The model under review builds one solid part; all positions refer to its coordinate system, in mm. Give positions to 0.01 mm unless a question says otherwise; leave off trailing zeros. Order: outer loops, then holes, each group sorted by start corner. A loop starts at its lowest first (then second) coordinate and runs counter-clockwise, first axis right, second up.
```python
from build123d import *

# Parameters (mm, degrees)
SKETCH1_R           = 75
SKETCH1_R_2         = 5
BOSS_EXTRUDE1_DEPTH = 5


with BuildPart() as part:
    # Sketch1 → Boss-Extrude1 (new, symmetric)
    with BuildSketch(Plane.XY):
        Circle(SKETCH1_R)
        with Locations((62.5, 0)):
            Circle(SKETCH1_R_2, mode=Mode.SUBTRACT)
        with Locations((54.126587737, -31.25)):
            Circle(SKETCH1_R_2, mode=Mode.SUBTRACT)
        with Locations((31.25, -54.126587737)):
            Circle(SKETCH1_R_2, mode=Mode.SUBTRACT)
        with Locations((0, -62.5)):
            Circle(SKETCH1_R_2, mode=Mode.SUBTRACT)
        with Locations((-31.25, -54.126587737)):
            Circle(SKETCH1_R_2, mode=Mode.SUBTRACT)
        with Locations((-54.126587737, -31.25)):
            Circle(SKETCH1_R_2, mode=Mode.SUBTRACT)
        with Locations((-62.5, 0)):
            Circle(SKETCH1_R_2, mode=Mode.SUBTRACT)
        with Locations((-54.126587737, 31.25)):
            Circle(SKETCH1_R_2, mode=Mode.SUBTRACT)
        with Locations((-31.25, 54.126587737)):
            Circle(SKETCH1_R_2, mode=Mode.SUBTRACT)
        with Locations((0, 62.5)):
            Circle(SKETCH1_R_2, mode=Mode.SUBTRACT)
        with Locations((31.25, 54.126587737)):
            Circle(SKETCH1_R_2, mode=Mode.SUBTRACT)
        with Locations((54.126587737, 31.25)):
            Circle(SKETCH1_R_2, mode=Mode.SUBTRACT)
        with BuildLine():
            Line((45, 5), (46.314144708, 5))
            ThreePointArc((46.314144708, 5), (48.608912113, 6.067632914), (49.27036671, 8.510638298))
            ThreePointArc((49.27036671, 8.510638298), (35.355339059, 35.355339059), (8.510638298, 49.27036671))
            ThreePointArc((8.510638298, 49.27036671), (6.067632914, 48.608912113), (5, 46.314144708))
            Line((5, 46.314144708), (5, 45))
            Line((5, 45), (-5, 45))
            Line((-5, 45), (-5, 46.314144708))
            ThreePointArc((-5, 46.314144708), (-6.067632914, 48.608912113), (-8.510638298, 49.27036671))
            ThreePointArc((-8.510638298, 49.27036671), (-35.355339059, 35.355339059), (-49.27036671, 8.510638298))
            ThreePointArc((-49.27036671, 8.510638298), (-48.608912113, 6.067632914), (-46.314144708, 5))
            Line((-46.314144708, 5), (-45, 5))
            Line((-45, 5), (-45, -5))
            Line((-45, -5), (-46.314144708, -5))
            ThreePointArc((-46.314144708, -5), (-48.608912113, -6.067632914), (-49.27036671, -8.510638298))
            ThreePointArc((-49.27036671, -8.510638298), (-35.355339059, -35.355339059), (-8.510638298, -49.27036671))
            ThreePointArc((-8.510638298, -49.27036671), (-6.067632914, -48.608912113), (-5, -46.314144708))
            Line((-5, -46.314144708), (-5, -45))
            Line((-5, -45), (5, -45))
            Line((5, -45), (5, -46.314144708))
            ThreePointArc((5, -46.314144708), (6.067632914, -48.608912113), (8.510638298, -49.27036671))
            ThreePointArc((8.510638298, -49.27036671), (35.355339059, -35.355339059), (49.27036671, -8.510638298))
            ThreePointArc((49.27036671, -8.510638298), (48.608912113, -6.067632914), (46.314144708, -5))
            Line((46.314144708, -5), (45, -5))
            Line((45, -5), (45, 5))
        make_face(mode=Mode.SUBTRACT)
    extrude(amount=BOSS_EXTRUDE1_DEPTH, both=True)


solid = part.part
```
Item 1: Clearance check with flat-ended pins moving along their axes: pin 1 Ø6 at (y, z) = (8.5, -1.5) entering from -X; pin 2 Ø1.1 at (x, z) = (-46, -1.5) entering from +Y; pin 3 Ø0.7 at (x, z) = (45.5, 1) entering from -Y; pin 4 Ø9 at (x, y) = (31.25, -54.13) entering from -Z. State where each tip first meets the part, or that it passes through.
Values found:
pin 1: stops at x = -74.8
pin 2: stops at y = 59.66
pin 3: stops at y = -59.89
pin 4: passes through
Item 2: Take a section at B-B (y = -62.5). Give the boundary of the cut face in (x, z), and give its area (3 significant figures).
Values found:
outline: (-41.46, -5) - (-5, -5) - (-5, 5) - (-41.46, 5) - close; (5, -5) - (41.46, -5) - (41.46, 5) - (5, 5) - close
area: 729 mm2
Item 3: Take a section at D-D (x = -63). Give the boundary of the cut face in (y, z).
Values found:
outline: (-40.69, -5) - (-4.97, -5) - (-4.97, 5) - (-40.69, 5) - close; (4.97, -5) - (40.69, -5) - (40.69, 5) - (4.97, 5) - close
Item 4: Take a section at A-A (x = 0). Give the boundary of the cut face in (y, z), and give its area (3 significant figures).
Values found:
outline: (-75, -5) - (-67.5, -5) - (-67.5, 5) - (-75, 5) - close; (-57.5, -5) - (-45, -5) - (-45, 5) - (-57.5, 5) - close; (45, -5) - (57.5, -5) - (57.5, 5) - (45, 5) - close; (67.5, -5) - (75, -5) - (75, 5) - (67.5, 5) - close
area: 400 mm2
Item 5: For line 1 (Y direction, x = 31.25, z = -2); line 2 (Y direction, x = -2, z = -2); line 3 (Y direction, x = 53.5, z = -4), list the stretches that pass through material, from the lowest coordinate up.
Values found:
line 1: y = -68.18 to -59.13, -49.13 to -39.03, 39.03 to 49.13, 59.13 to 68.18
line 2: y = -74.97 to -67.08, -57.92 to -45, 45 to 57.92, 67.08 to 74.97
line 3: y = -52.56 to -36.21, -26.29 to 26.29, 36.21 to 52.56
Item 6: Draft analysis for pull direction Y (two halves, no side actions). For faces 1 (the cylindrical face through (50.159, -34.292, -0.07)), 2 (the flat face through (-1, -49, 5)), state which applies: released by +Y, released by -Y, zero draft, split by the parting line, or undercut.
Values found:
face 1: undercut
face 2: zero draft
